```python
from build123d import *

# Parameters (mm, degrees)
EXTRUDE_1_DEPTH                = 50
SPLIT_BODIES_1_SURFACE_1_BACK  = 226.829
SPLIT_BODIES_1_SURFACE_1_DEPTH = 453.658
SPLIT_BODIES_1_SURFACE_2_BACK  = 226.829
SPLIT_BODIES_1_SURFACE_2_DEPTH = 453.658


with BuildPart() as part:
    # 草图2 → 凸台-拉伸1 (new, symmetric)
    with BuildSketch(Plane.XY):
        with BuildLine():
            Line((120.381757685, 47.561632043), (136.603924057, 47.561632043))
            Line((136.603924057, 47.561632043), (146.850265064, 88.947420909))
            ThreePointArc((146.850265064, 88.947420909), (104.62030332, 85.070472378), (109.988846824, 127.136838271))
            Line((109.988846824, 127.136838271), (88.280849451, 128.197534042))
            ThreePointArc((88.280849451, 128.197534042), (80.571822415, 123.964886157), (80.863683371, 115.175163571))
            ThreePointArc((80.863683371, 115.175163571), (88.300101913, 100.587398022), (92.288223879, 84.706651578))
            Line((92.288223879, 84.706651578), (52.259104564, 84.706651578))
            Line((52.259104564, 84.706651578), (52.259104564, 37.347972633))
            Line((52.259104564, 37.347972633), (26.12059868, 28.530814049))
            Line((26.12059868, 28.530814049), (0, 28.530814049))
            Line((0, 28.530814049), (0, 0))
            Line((0, 0), (140.98, 0))
            Line((140.98, 0), (131.928221984, 26.834036233))
            Line((131.928221984, 26.834036233), (115.249995775, 26.834036233))
            Line((115.249995775, 26.834036233), (120.381757685, 47.561632043))
        make_face()
        with BuildLine():
            ThreePointArc((109.988846824, 127.136838271), (104.62030332, 85.070472378), (146.850265064, 88.947420909))
            Line((146.850265064, 88.947420909), (151.231226865, 106.642475172))
            ThreePointArc((151.231226865, 106.642475172), (147.884639105, 117.258207331), (140.564064785, 125.64287253))
            Line((140.564064785, 125.64287253), (109.988846824, 127.136838271))
        make_face()
        with BuildLine():
            ThreePointArc((140.564064785, 125.64287253), (125.506724817, 131.102497099), (109.988846824, 127.136838271))
            Line((109.988846824, 127.136838271), (140.564064785, 125.64287253))
        make_face()
        with BuildLine():
            ThreePointArc((140.564064785, 125.64287253), (147.884639105, 117.258207331), (151.231226865, 106.642475172))
            Line((151.231226865, 106.642475172), (154.115877694, 118.293810031))
            ThreePointArc((154.115877694, 118.293810031), (153.172952645, 122.982290954), (148.95330104, 125.232957822))
            Line((148.95330104, 125.232957822), (140.564064785, 125.64287253))
        make_face()
    extrude(amount=EXTRUDE_1_DEPTH, both=True)


with BuildPart() as body_2:
    # Split Bodies 1: the piece behind the surface
    add(part.part)
    # Split Bodies 1 surface: a surface, the sketch's curves swept straight by 453.658 mm
    with BuildLine(Plane.XY.offset(50).offset(-SPLIT_BODIES_1_SURFACE_1_BACK), mode=Mode.PRIVATE) as split_bodies_1_surface_1_path:
        Line((120.381757685, 47.561632043), (52.259104564, 47.561632043))
    split_bodies_1_surface_1 = Shell.extrude(split_bodies_1_surface_1_path.wire(), (0 * SPLIT_BODIES_1_SURFACE_1_DEPTH, 0 * SPLIT_BODIES_1_SURFACE_1_DEPTH, 1 * SPLIT_BODIES_1_SURFACE_1_DEPTH))
    split(bisect_by=split_bodies_1_surface_1, keep=Keep.BOTTOM)


with BuildPart() as part_1:
    add(part.part)

    # Split Bodies 1: split by a surface, the side it looks to stays
    # Split Bodies 1 surface: a surface, the sketch's curves swept straight by 453.658 mm
    with BuildLine(Plane.XY.offset(50).offset(-SPLIT_BODIES_1_SURFACE_2_BACK), mode=Mode.PRIVATE) as split_bodies_1_surface_2_path:
        Line((120.381757685, 47.561632043), (52.259104564, 47.561632043))
    split_bodies_1_surface_2 = Shell.extrude(split_bodies_1_surface_2_path.wire(), (0 * SPLIT_BODIES_1_SURFACE_2_DEPTH, 0 * SPLIT_BODIES_1_SURFACE_2_DEPTH, 1 * SPLIT_BODIES_1_SURFACE_2_DEPTH))
    split(bisect_by=split_bodies_1_surface_2, keep=Keep.TOP)


solid = part_1.part
```
CAD build for the part. Positions are in the model's coordinates, mm. A direction names the side the tool comes from. Coordinates: 2 decimals unless noted, no trailing zeros. Write each loop counter-clockwise with the first axis right and the second up, starting at its lowest first coordinate (ties: lowest second). Pieces come first, ordered by that corner, then holes. Notation, with made-up numbers: (6, 44) -> (48, 44) arc R17 cw to (48, 69) -> close; hole circle Ø9 at (89.5, -19.75). An arc over 180 degrees is marked (long way). Return JSON: item names as keys, results as strings. Group by question number.
Q1. Cut at B-B, the plane x = 19. Give the cut face in (y, z), then the cut area to 3 significant figures.
Q2. Cut at A-A, the plane z = -32.5. Give the cut face in (x, y), then the cut area to 3 significant figures.
Q3. Cut at C-C, the plane y = 30. Give the cut face in (x, z), then the cut area to 3 significant figures.
Q4. Which spindle directions (+Z, -Z, +X, -X, +Y, -Y) get a long thin tool onto all of the face, cutting with end or side? Do faces 1 (the face through (52.259, 43, 1)), 2 (the face through (136.517, 13.229, 0.7)). Say none if no direction does.
Q5. Pull direction Y, two halves, no side cores. Call faces 3 (the face through (124, 26.834, 1)), 4 (the face through (117.78, 37.05, 0.7)), 5 (the face through (39.37, 33, 0.7)), 6 (the face through (70, 19, 50)): released by +Y, released by -Y, zero draft, split by the parting line, or undercut.
Q6. Drill centre lines: line 1 (Y direction, x = 22.5, z = 43); line 2 (X direction, y = 22, z = 42); line 3 (X direction, y = 3.5, z = 24.5). Where is each one in solid material? Low to high.
Q7. Flat gauge pins, fed straight in: pin 1 (8 mm diameter, centred on y = 42.5, z = 2, fed in from -X); pin 2 (6 mm diameter, centred on y = 26, z = -2.5, fed in from -X); pin 3 (12 mm diameter, centred on y = 12, z = -16, fed in from +X); pin 4 (5 mm diameter, centred on x = 124, z = 5.5, fed in from +Y). Where does each tip first touch, or does it go through?
Returned:
{
 "1": {"outline": "(0, -50) -> (28.53, -50) -> (28.53, 50) -> (0, 50) -> close", "area": "2,850 mm2"},
 "2": {"outline": "(0, 0) -> (140.98, 0) -> (131.93, 26.83) -> (115.25, 26.83) -> (120.38, 47.56) -> (52.26, 47.56) -> (52.26, 37.35) -> (26.12, 28.53) -> (0, 28.53) -> close", "area": "5,220 mm2"},
 "3": {"outline": "(30.48, -50) -> (116.03, -50) -> (116.03, 50) -> (30.48, 50) -> close", "area": "8,560 mm2"},
 "4": {"face 1": "+Z, -Z, -X, +Y", "face 2": "+Z, -Z, +X, +Y"},
 "5": {"face 3": "undercut", "face 4": "undercut", "face 5": "released by +Y", "face 6": "zero draft"},
 "6": {"line 1": "y = 0 to 28.53", "line 2": "x = 0 to 133.56", "line 3": "x = 0 to 139.8"},
 "7": {"pin 1": "stops at x = 52.26", "pin 2": "stops at x = 0", "pin 3": "stops at x = 138.96", "pin 4": "stops at y = 26.83"}
}
